Read the model definition and answer for the solid it produces. Units are mm, in the model's axes. A direction names the side the tool comes from. Round coordinates to 2 decimals unless told otherwise and drop trailing zeros. Order: outer loops, then holes, each group sorted by start corner. A loop starts at its lowest first (then second) coordinate and runs counter-clockwise, first axis right, second up. Notation, with made-up numbers: (48.25, -19.5) -> (73.25, -19.5) arc R18 ccw to (73.25, 14.5) -> close; hole circle Ø5 at (20, -24). An arc over 180 degrees is marked (long way). Use a Markdown table: item, result. Add a question column.
1. Section C-C, the plane z = -17.5 is taken. Give the vertices of the cut face in (x, y), then the cut area to 3 significant figures.
2. Section A-A, the plane x = -13.5 is taken. Give the vertices of the cut face in (y, z), then the cut area to 3 significant figures.
3. For faces 1 (the face through (3.604, -10.846, -11.446)), 2 (the face through (-5, 3, 10)), 3 (the face through (-8.618, 1.479, 20.784)), determine the directions among +Z, -Z, +X, -X, +Y, -Y from which every point of the face is accessible in a straight line to the end or side of a thin tool.
4. Consider L1, parallel to Y at x = 13.5, z = 3; L2, parallel to X at y = 14, z = 8; L3, parallel to Z at x = -4, y = -13.5. Determine where each line is inside the solid, lowest interval first. Write a range as [from, to].
5. Section B-B, the plane y = 15 is taken. Give the vertices of the cut face in (x, z), then the cut area to 3 significant figures.
6. Section D-D, the plane y = -11 is taken. Give the vertices of the cut face in (x, z), then the cut area to 3 significant figures.
7. Given pin 1 (4 mm diameter, centred on y = 20.5, z = -3.5, fed in from -X); pin 2 (13.5 mm diameter, centred on x = -11, z = 7.5, fed in from -Y); pin 3 (10 mm diameter, centred on x = 2.5, y = 19.5, fed in from +Z), each flat-ended and moving along its own axis, determine where each tip first touches the part or whether it passes through.
```python
from build123d import *

# Parameters (mm, degrees)
SKETCH1_R           = 22.5
BOSS_EXTRUDE3_DEPTH = 3
SKETCH2_R           = 10
BOSS_EXTRUDE5_DEPTH = 70
SKETCH5_R           = 12
BOSS_EXTRUDE6_DEPTH = 28
FILLET1_R           = 6


with BuildPart() as part:
    # Sketch1 → Boss-Extrude3 (new body)
    with BuildSketch(Plane(origin=(0, 0, 0), x_dir=(1, 0, 0), z_dir=(0, 1, 0))):
        with Locations(Location((0, 0, 0), (0, 0, 270))):
            Circle(SKETCH1_R)
    extrude(amount=BOSS_EXTRUDE3_DEPTH)

    # Sketch2 → Boss-Extrude5 (add)
    with BuildSketch(Plane(origin=(0, 3, 0), x_dir=(1, 0, 0), z_dir=(0, 1, 0))):
        with Locations(Location((0, 0, 0), (0, 0, 270))):
            Circle(SKETCH2_R)
    extrude(amount=BOSS_EXTRUDE5_DEPTH)

    # Sketch5 → Boss-Extrude6 (add)
    with BuildSketch(Plane.XZ):
        with Locations(Location((0, 0, 0), (0, 0, 270))):
            Circle(SKETCH5_R)
    extrude(amount=BOSS_EXTRUDE6_DEPTH)

    # Fillet1
    fillet1_edges = [part.edges().sort_by_distance(p)[0] for p in [
        (0, -28, 12),
    ]]
    fillet(fillet1_edges, radius=FILLET1_R)


solid = part.part
```
Verdict:
| question | item | result |
|---|---|---|
| 1 | outline | (-14.14, 0) -> (14.14, 0) -> (14.14, 3) -> (-14.14, 3) -> close |
| 1 | area | 84.9 mm2 |
| 2 | outline | (0, -18) -> (3, -18) -> (3, 18) -> (0, 18) -> close |
| 2 | area | 108 mm2 |
| 3 | face 1 | -Y |
| 3 | face 2 | +Y |
| 3 | face 3 | +Y, -Y |
| 4 | L1 | y = [0, 3] |
| 4 | L2 | x = [-6, 6] |
| 4 | L3 | z = [-11.31, 11.31] |
| 5 | outline | circle Ø20 at (0, 0) |
| 5 | area | 314 mm2 |
| 6 | outline | circle Ø24 at (0, 0) |
| 6 | area | 452 mm2 |
| 7 | pin 1 | stops at x = -9.89 |
| 7 | pin 2 | stops at y = -27.97 |
| 7 | pin 3 | stops at z = 10 |
